The listing builds one solid part. Answer for the finished solid, in the listing's coordinates (mm). Face numbers are marked on the shaded views. A direction names the side the tool comes from. Round coordinates to 2 decimals unless told otherwise and drop trailing zeros. Order: outer loops, then holes, each group sorted by start corner. A loop starts at its lowest first (then second) coordinate and runs counter-clockwise, first axis right, second up. Notation, with made-up numbers: (-2, -10) - (54, -10) arc R36 ccw to (54, 24) - close; hole circle Ø7 at (75.25, 83.5). An arc over 180 degrees is marked (long way). Use CSV: the item, a comma, the result in double quotes. Start each with the question number.
Item 1: Determine the mould class of the marked faces 1, 2 and 3 for opening direction X: +X half, -X half, draft (parallel to the pull), parting line (faces both ways), or undercut.
Item 2: For the marked faces 4, 5 and 6, determine the directions among +Z, -Z, +X, -X, +Y, -Y from which every point of the face is accessible in a straight line to the end or side of a thin tool.
Item 3: Straight lines are drawn through the part: line 1 along X through (y, z) = (3.45, 0); line 2 along X through (y, z) = (3.7, 3); line 3 along X through (y, z) = (3.5, -7). For each, find the intervals that lie inside material, in ascending order. Write a range as [from, to].
Item 4: Find section C-C, the plane z = -7. Give the vertices of the cut face in (x, y).
Item 5: Find section B-B, the plane x = -3.75. Give the vertices of the cut face in (y, z).
Item 6: Flat-ended cylindrical pins translate along their axes: P1, Ø2.5, axis at x = 7, z = 0, coming from the -Y side; P2, Ø2, axis at y = 3, z = -6.5, coming from the +X side; P3, Ø3, axis at x = 0, z = -0.5, coming from the +Y side. Find the tip coordinate at first contact, or state that the pin passes through.
Item 7: Find section A-A, the plane y = 4.35. Count the separate pieces of the cut face and the enclosed holes in it, plus the area to 3 significant figures.
```python
from build123d import *

# Parameters (mm, degrees)
SKETCH1_R           = 4
SKETCH1_R_2         = 3
BOSS_EXTRUDE1_DEPTH = 3
SKETCH2_R           = 10
BOSS_EXTRUDE2_DEPTH = 2
CUT_EXTRUDE1_REACH  = 17
SKETCH3_R           = 1
SKETCH3_R_2         = 1.5
SKETCH4_R           = 4.5
SKETCH4_R_2         = 3.2
SKETCH4_R_3         = 3
SKETCH4_R_4         = 1.5
CUT_EXTRUDE2_DEPTH  = 1


with BuildPart() as part:
    # Sketch1 → Boss-Extrude1 (new body)
    with BuildSketch(Plane(origin=(0, 0, 0), x_dir=(1, 0, 0), z_dir=(0, 1, 0))):
        with Locations(Location((0, 0, 0), (0, 0, 270))):
            Circle(SKETCH1_R)
        with Locations(Location((0, 0, 0), (0, 0, 270))):
            Circle(SKETCH1_R_2, mode=Mode.SUBTRACT)
    extrude(amount=BOSS_EXTRUDE1_DEPTH)

    # Sketch2 → Boss-Extrude2 (add)
    with BuildSketch(Plane(origin=(0, 3, 0), x_dir=(1, 0, 0), z_dir=(0, 1, 0))):
        with Locations(Location((0, 0, 0), (0, 0, 270))):
            Circle(SKETCH2_R)
    extrude(amount=BOSS_EXTRUDE2_DEPTH)

    # Sketch3 → Cut-Extrude1 (cut, up to next)
    with BuildSketch(Plane(origin=(0, 5, 0), x_dir=(1, 0, 0), z_dir=(0, 1, 0)), mode=Mode.PRIVATE) as cut_extrude1_sk1:
        with Locations(Location((0, 7, 0), (0, 0, 270))):
            Circle(SKETCH3_R)
    cut_extrude1_tool1 = extrude(cut_extrude1_sk1.sketch, amount=-CUT_EXTRUDE1_REACH, mode=Mode.PRIVATE) & part.part
    # Sketch3 → Cut-Extrude1 (cut, up to next)
    with BuildSketch(Plane(origin=(0, 5, 0), x_dir=(1, 0, 0), z_dir=(0, 1, 0)), mode=Mode.PRIVATE) as cut_extrude1_sk2:
        with Locations(Location((3, 7, 0), (0, 0, 270))):
            Circle(SKETCH3_R)
    cut_extrude1_tool2 = extrude(cut_extrude1_sk2.sketch, amount=-CUT_EXTRUDE1_REACH, mode=Mode.PRIVATE) & part.part
    # Sketch3 → Cut-Extrude1 (cut, up to next)
    with BuildSketch(Plane(origin=(0, 5, 0), x_dir=(1, 0, 0), z_dir=(0, 1, 0)), mode=Mode.PRIVATE) as cut_extrude1_sk3:
        with Locations(Location((-3, 7, 0), (0, 0, 270))):
            Circle(SKETCH3_R)
    cut_extrude1_tool3 = extrude(cut_extrude1_sk3.sketch, amount=-CUT_EXTRUDE1_REACH, mode=Mode.PRIVATE) & part.part
    # Sketch3 → Cut-Extrude1 (cut, up to next)
    with BuildSketch(Plane(origin=(0, 5, 0), x_dir=(1, 0, 0), z_dir=(0, 1, 0)), mode=Mode.PRIVATE) as cut_extrude1_sk4:
        with Locations(Location((7, 3, 0), (0, 0, 270))):
            Circle(SKETCH3_R)
    cut_extrude1_tool4 = extrude(cut_extrude1_sk4.sketch, amount=-CUT_EXTRUDE1_REACH, mode=Mode.PRIVATE) & part.part
    # Sketch3 → Cut-Extrude1 (cut, up to next)
    with BuildSketch(Plane(origin=(0, 5, 0), x_dir=(1, 0, 0), z_dir=(0, 1, 0)), mode=Mode.PRIVATE) as cut_extrude1_sk5:
        with Locations(Location((7, 0, 0), (0, 0, 270))):
            Circle(SKETCH3_R)
    cut_extrude1_tool5 = extrude(cut_extrude1_sk5.sketch, amount=-CUT_EXTRUDE1_REACH, mode=Mode.PRIVATE) & part.part
    # Sketch3 → Cut-Extrude1 (cut, up to next)
    with BuildSketch(Plane(origin=(0, 5, 0), x_dir=(1, 0, 0), z_dir=(0, 1, 0)), mode=Mode.PRIVATE) as cut_extrude1_sk6:
        with Locations(Location((7, -3, 0), (0, 0, 270))):
            Circle(SKETCH3_R)
    cut_extrude1_tool6 = extrude(cut_extrude1_sk6.sketch, amount=-CUT_EXTRUDE1_REACH, mode=Mode.PRIVATE) & part.part
    # Sketch3 → Cut-Extrude1 (cut, up to next)
    with BuildSketch(Plane(origin=(0, 5, 0), x_dir=(1, 0, 0), z_dir=(0, 1, 0)), mode=Mode.PRIVATE) as cut_extrude1_sk7:
        with Locations(Location((3, -7, 0), (0, 0, 270))):
            Circle(SKETCH3_R)
    cut_extrude1_tool7 = extrude(cut_extrude1_sk7.sketch, amount=-CUT_EXTRUDE1_REACH, mode=Mode.PRIVATE) & part.part
    # Sketch3 → Cut-Extrude1 (cut, up to next)
    with BuildSketch(Plane(origin=(0, 5, 0), x_dir=(1, 0, 0), z_dir=(0, 1, 0)), mode=Mode.PRIVATE) as cut_extrude1_sk8:
        with Locations(Location((0, -7, 0), (0, 0, 270))):
            Circle(SKETCH3_R)
    cut_extrude1_tool8 = extrude(cut_extrude1_sk8.sketch, amount=-CUT_EXTRUDE1_REACH, mode=Mode.PRIVATE) & part.part
    # Sketch3 → Cut-Extrude1 (cut, up to next)
    with BuildSketch(Plane(origin=(0, 5, 0), x_dir=(1, 0, 0), z_dir=(0, 1, 0)), mode=Mode.PRIVATE) as cut_extrude1_sk9:
        with Locations(Location((-3, -7, 0), (0, 0, 270))):
            Circle(SKETCH3_R)
    cut_extrude1_tool9 = extrude(cut_extrude1_sk9.sketch, amount=-CUT_EXTRUDE1_REACH, mode=Mode.PRIVATE) & part.part
    # Sketch3 → Cut-Extrude1 (cut, up to next)
    with BuildSketch(Plane(origin=(0, 5, 0), x_dir=(1, 0, 0), z_dir=(0, 1, 0)), mode=Mode.PRIVATE) as cut_extrude1_sk10:
        with Locations(Location((-7, -3, 0), (0, 0, 270))):
            Circle(SKETCH3_R)
    cut_extrude1_tool10 = extrude(cut_extrude1_sk10.sketch, amount=-CUT_EXTRUDE1_REACH, mode=Mode.PRIVATE) & part.part
    # Sketch3 → Cut-Extrude1 (cut, up to next)
    with BuildSketch(Plane(origin=(0, 5, 0), x_dir=(1, 0, 0), z_dir=(0, 1, 0)), mode=Mode.PRIVATE) as cut_extrude1_sk11:
        with Locations(Location((-7, 0, 0), (0, 0, 270))):
            Circle(SKETCH3_R)
    cut_extrude1_tool11 = extrude(cut_extrude1_sk11.sketch, amount=-CUT_EXTRUDE1_REACH, mode=Mode.PRIVATE) & part.part
    # Sketch3 → Cut-Extrude1 (cut, up to next)
    with BuildSketch(Plane(origin=(0, 5, 0), x_dir=(1, 0, 0), z_dir=(0, 1, 0)), mode=Mode.PRIVATE) as cut_extrude1_sk12:
        with Locations(Location((-7, 3, 0), (0, 0, 270))):
            Circle(SKETCH3_R)
    cut_extrude1_tool12 = extrude(cut_extrude1_sk12.sketch, amount=-CUT_EXTRUDE1_REACH, mode=Mode.PRIVATE) & part.part
    # Sketch3 → Cut-Extrude1 (cut, up to next)
    with BuildSketch(Plane(origin=(0, 5, 0), x_dir=(1, 0, 0), z_dir=(0, 1, 0)), mode=Mode.PRIVATE) as cut_extrude1_sk13:
        with Locations(Location((0, 0, 0), (0, 0, 270))):
            Circle(SKETCH3_R_2)
    cut_extrude1_tool13 = extrude(cut_extrude1_sk13.sketch, amount=-CUT_EXTRUDE1_REACH, mode=Mode.PRIVATE) & part.part
    add(cut_extrude1_tool1.solids().sort_by_distance((0, 5, -7))[0], mode=Mode.SUBTRACT)
    add(cut_extrude1_tool2.solids().sort_by_distance((3, 5, -7))[0], mode=Mode.SUBTRACT)
    add(cut_extrude1_tool3.solids().sort_by_distance((-3, 5, -7))[0], mode=Mode.SUBTRACT)
    add(cut_extrude1_tool4.solids().sort_by_distance((7, 5, -3))[0], mode=Mode.SUBTRACT)
    add(cut_extrude1_tool5.solids().sort_by_distance((7, 5, 0))[0], mode=Mode.SUBTRACT)
    add(cut_extrude1_tool6.solids().sort_by_distance((7, 5, 3))[0], mode=Mode.SUBTRACT)
    add(cut_extrude1_tool7.solids().sort_by_distance((3, 5, 7))[0], mode=Mode.SUBTRACT)
    add(cut_extrude1_tool8.solids().sort_by_distance((0, 5, 7))[0], mode=Mode.SUBTRACT)
    add(cut_extrude1_tool9.solids().sort_by_distance((-3, 5, 7))[0], mode=Mode.SUBTRACT)
    add(cut_extrude1_tool10.solids().sort_by_distance((-7, 5, 3))[0], mode=Mode.SUBTRACT)
    add(cut_extrude1_tool11.solids().sort_by_distance((-7, 5, 0))[0], mode=Mode.SUBTRACT)
    add(cut_extrude1_tool12.solids().sort_by_distance((-7, 5, -3))[0], mode=Mode.SUBTRACT)
    add(cut_extrude1_tool13.solids().sort_by_distance((0, 5, 0))[0], mode=Mode.SUBTRACT)

    # Sketch4 → Cut-Extrude2 (cut)
    # profile 1 of 2: a face of its own
    with BuildSketch(Plane(origin=(0, 5, 0), x_dir=(1, 0, 0), z_dir=(0, 1, 0))):
        with Locations(Location((0, 0, 0), (0, 0, 270))):
            Circle(SKETCH4_R)
        with Locations(Location((0, 0, 0), (0, 0, 270))):
            Circle(SKETCH4_R_2, mode=Mode.SUBTRACT)
    # profile 2 of 2: a face of its own
    with BuildSketch(Plane(origin=(0, 5, 0), x_dir=(1, 0, 0), z_dir=(0, 1, 0))):
        with Locations(Location((0, 0, 0), (0, 0, 270))):
            Circle(SKETCH4_R_3)
        with Locations(Location((0, 0, 0), (0, 0, 270))):
            Circle(SKETCH4_R_4, mode=Mode.SUBTRACT)
    extrude(amount=-CUT_EXTRUDE2_DEPTH, mode=Mode.SUBTRACT)


solid = part.part
```
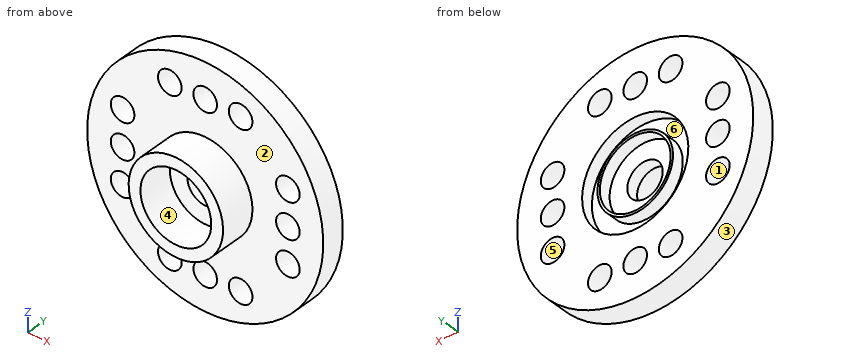
Worked out:
1,face 1,"undercut"
1,face 2,"draft"
1,face 3,"parting line"
2,face 4,"-Y"
2,face 5,"+Y, -Y"
2,face 6,"+Y"
3,line 1,"x = [-10, -8], [-6, -1.5], [1.5, 6], [8, 10]"
3,line 2,"x = [-9.54, -8], [-6, 6], [8, 9.54]"
3,line 3,"x = [-7.14, -4], [-2, -1], [1, 2], [4, 7.14]"
4,outline,"(-7.14, 3) - (-4, 3) - (-4, 5) - (-7.14, 5) - close; (-2, 3) - (-1, 3) - (-1, 5) - (-2, 5) - close; (1, 3) - (2, 3) - (2, 5) - (1, 5) - close; (4, 3) - (7.14, 3) - (7.14, 5) - (4, 5) - close"
5,outline,"(0, -1.39) - (3, -1.39) - (3, -6.34) - (5, -6.34) - (5, -2.49) - (4, -2.49) - (4, 2.49) - (5, 2.49) - (5, 6.34) - (3, 6.34) - (3, 1.39) - (0, 1.39) - close; (3, -9.27) - (5, -9.27) - (5, -7.66) - (3, -7.66) - close; (3, 7.66) - (5, 7.66) - (5, 9.27) - (3, 9.27) - close"
6,P1,"stops at y = 3"
6,P2,"stops at x = 8.35"
6,P3,"stops at y = 4"
7,separate pieces,"2"
7,enclosed holes,"14"
7,area,"217 mm²"
